The listing builds one solid part. Answer for the finished solid, in the listing's coordinates (mm). Face numbers are marked on the shaded views. Give positions to 0.01 mm unless a question says otherwise; leave off trailing zeros. Order: outer loops, then holes, each group sorted by start corner. A loop starts at its lowest first (then second) coordinate and runs counter-clockwise, first axis right, second up. Notation, with made-up numbers: (80.25, -7) -> (103.25, -7) arc R24 cw to (103.25, 21) -> close; hole circle Ø1 at (40.25, 61.5). An arc over 180 degrees is marked (long way). One line per question, with ' | ' between items. Start each with the question number.
Autodesk Inventor part; units mm, degrees
ref_plane "YZ Plane" through (0, 0, 0) normal (1, 0, 0) x (0, 1, 0)
ref_plane "XZ Plane" through (0, 0, 0) normal (0, 1, 0) x (-1, 0, 0)
ref_plane "XY Plane" through (0, 0, 0) normal (0, 0, 1) x (1, 0, 0)
sketch "Sketch1" plane through (0, 0, 0) normal (0, 1, 0) x (-1, 0, 0)
  circle A0 centre (0, 0) radius 15
  dimension "d0" = 30
extrude "Extrusion1" add sketch "Sketch1" along normal blind 5
sketch "Sketch2" plane through (0, 5, 0) normal (0, 1, 0) x (1, 0, 0)
  circle A0 centre (0, 0) radius 7.5
  dimension "d3" = 15
extrude "Extrusion2" add sketch "Sketch2" along normal blind 5
sketch "Sketch3" plane through (0, 10, 0) normal (0, 1, 0) x (1, 0, 0)
  circle A0 centre (0, 0) radius 15
  dimension "d6" = 30
extrude "Extrusion3" add sketch "Sketch3" along normal blind 5
fillet "Fillet1" radius 3.175 1 edges at (-15, 15, 0)
fillet "Fillet2" radius 3.175 1 edges at (-15, 10, 0)
fillet "Fillet3" radius 3.175 1 edges at (-7.5, 10, 0)
fillet "Fillet4" radius 3.175 1 edges at (15, 5, 0)
fillet "Fillet5" radius 3.175 1 edges at (15, 0, 0)
fillet "Fillet6" radius 3.175 1 edges at (-7.5, 5, 0)
hole "Hole1" at (0, 15, 0) direction (0, -1, 0) diameter 5 end through all
properties part number "even more awesome inventor thing"
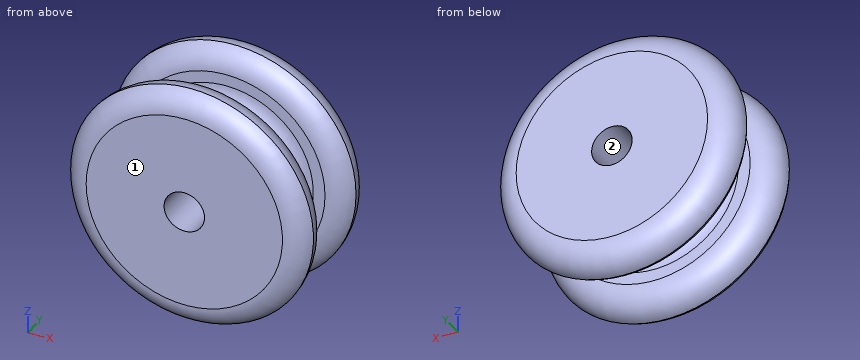
(1) The part is cut by section D-D on y = 12.75. Determine the outline of the cut face in (x, z), plus the area to 3 significant figures.
(2) Consider line 1 (Y direction, x = -10, z = -6); line 2 (Z direction, x = 0, y = 12); line 3 (X direction, y = 6.25, z = 0). Determine where each line is inside the solid, lowest interval first.
(3) The part is cut by section C-C on y = 8.5. Determine the outline of the cut face in (x, z), plus the area to 3 significant figures.
(4) Determine the mould class of the marked faces 1 and 2 for opening direction X: pulls with the +X half, pulls with the -X half, needs draft (parallel to the pull), parting line crosses it, or undercut.
(5) The part is cut by section A-A on z = 0. Determine the outline of the cut face in (x, y) (3 decimals), plus the area to 3 significant figures.
(6) Given P1, Ø1.5, axis at x = -3, y = 9.5, coming from the +Z side; P2, Ø2, axis at x = 11.5, y = 2.5, coming from the -Z side; P3, Ø6, axis at x = -4.5, y = 12.5, coming from the +Z side; P4, Ø5, axis at y = 12, z = -1, coming from the -X side, each flat-ended and moving along its own axis, determine where each tip first touches the part or whether it passes through.
(7) The part is cut by section B-B on x = 0. Determine the outline of the cut face in (y, z) (3 decimals), plus the area to 3 significant figures.
Result sheet:
1) outline: circle Ø29.72 at (0, 0); hole circle Ø5 at (0, 0) | area: 674 mm^2
2) line 1: y = 0 to 5, 10 to 15 | line 2: z = -15 to -2.5, 2.5 to 15 | line 3: x = -7.85 to -2.5, 2.5 to 7.85
3) outline: circle Ø15.96 at (0, 0); hole circle Ø5 at (0, 0) | area: 180 mm^2
4) face 1: needs draft | face 2: undercut
5) outline: (-15, 1.825) arc R3.175 ccw to (-12.126, 0) -> (-2.5, 0) -> (-2.5, 15) -> (-11.825, 15) arc R3.175 ccw to (-15, 11.825) arc R3.175 ccw to (-12.126, 10) -> (-10.675, 10) arc R3.175 cw to (-7.5, 6.825) arc R3.175 cw to (-10.374, 5) -> (-11.825, 5) arc R3.175 ccw to start; (2.5, 0) -> (12.126, 0) arc R3.175 ccw to (15, 1.825) arc R3.175 ccw to (11.825, 5) -> (10.374, 5) arc R3.175 cw to (7.5, 6.825) arc R3.175 cw to (10.675, 10) -> (12.126, 10) arc R3.175 ccw to (15, 11.825) arc R3.175 ccw to (11.825, 15) -> (2.5, 15) -> close | area: 293 mm^2
6) P1: stops at z = 13.03 | P2: stops at z = -10.64 | P3: stops at z = 14.92 | P4: stops at x = -15
7) outline: (0, -12.126) arc R3.175 ccw to (1.825, -15) arc R3.175 ccw to (5, -11.825) -> (5, -10.374) arc R3.175 cw to (6.825, -7.5) arc R3.175 cw to (10, -10.675) -> (10, -12.126) arc R3.175 ccw to (11.825, -15) arc R3.175 ccw to (15, -11.825) -> (15, -2.5) -> (0, -2.5) -> close; (0, 2.5) -> (15, 2.5) -> (15, 11.825) arc R3.175 ccw to (11.825, 15) arc R3.175 ccw to (10, 12.126) -> (10, 10.675) arc R3.175 cw to (6.825, 7.5) arc R3.175 cw to (5, 10.374) -> (5, 11.825) arc R3.175 ccw to (1.825, 15) arc R3.175 ccw to (0, 12.126) -> close | area: 293 mm^2
